Design review of the part built by this model. Coordinates are the model's own, in mm. A direction names the side the tool comes from. Give positions to 0.01 mm unless a question says otherwise; leave off trailing zeros. Loops run counter-clockwise (first coordinate to the right, second up) from the corner with the lowest first, then second, coordinate; pieces in that order, holes last. Notation, with made-up numbers: M -4.75,-22.75 L 8.25,-22.75 A21 ccw 8.25,3.25 Z; hole C 52,0.25 d5. An arc over 180 degrees is marked long. Use a Markdown table: item, result. Add a question column.
(1) Insertion check: pin 1 Ø3 at (x, y) = (-1, 56) entering from -Z; pin 2 Ø8 at (y, z) = (14.5, -5.5) entering from -X. Each pin has a flat end and moves straight along its axis. Give the tip position at first contact, or say it passes through.
(2) Add section B-B, the plane y = 42. Give the boundary of the cut face in (x, z).
(3) For faces 1 (the face through (-0.867, 31.798, 3.905)), 2 (the face through (-2.5, 67, 6)), list the 3-axis set-ups (+Z, -Z, +X, -X, +Y, -Y) from which the entire face can be reached by the end or side of a thin tool; tool diameter is ignored.
(4) Add section A-A, the plane z = -2.5. Give the boundary of the cut face in (x, y), then the cut area to 3 significant figures.
(5) Add section C-C, the plane z = 5.75. Give the boundary of the cut face in (x, y).
(6) For probe 1 along Z at (x, y) = (0.25, 23); probe 2 along Y at (x, z) = (-4.25, 2.75); probe 3 along X at (y, z) = (14, -0.5), list the stretches that pass through material, from the lowest coordinate up.
```python
from build123d import *

# Parameters (mm, degrees)
SKETCH1_R           = 4
BOSS_EXTRUDE1_DEPTH = 64.5
BOSS_EXTRUDE2_DEPTH = 5
CHAMFER1_SIZE       = 0.65


with BuildPart() as part:
    # Sketch1 → Boss-Extrude1 (new body)
    with BuildSketch(Plane(origin=(0, 0, 0), x_dir=(1, 0, 0), z_dir=(0, 1, 0))):
        Circle(SKETCH1_R)
    extrude(amount=BOSS_EXTRUDE1_DEPTH)

    # Sketch2 → Boss-Extrude2 (add)
    with BuildSketch(Plane(origin=(0, 64.5, 0), x_dir=(1, 0, 0), z_dir=(0, 1, 0))):
        Polygon((7.035549302, 0), (4.974884621, 4.974884621), (0, 7.035549302), (-4.974884621, 4.974884621), (-7.035549302, 0), (-4.974884621, -4.974884621), (0, -7.035549302), (4.974884621, -4.974884621), align=None)
    extrude(amount=BOSS_EXTRUDE2_DEPTH)

    # Chamfer1
    chamfer1_edges = [part.edges().sort_by_distance(p)[0] for p in [
        (-6.005216961, 69.5, 2.48744231),
        (-2.48744231, 69.5, 6.005216961),
        (2.48744231, 69.5, 6.005216961),
        (6.005216961, 64.5, 2.48744231),
        (6.005216961, 64.5, -2.48744231),
        (2.48744231, 64.5, -6.005216961),
        (-2.48744231, 64.5, -6.005216961),
        (-6.005216961, 64.5, -2.48744231),
        (-6.005216961, 64.5, 2.48744231),
        (-2.48744231, 64.5, 6.005216961),
        (2.48744231, 64.5, 6.005216961),
        (6.005216961, 69.5, 2.48744231),
        (6.005216961, 69.5, -2.48744231),
        (2.48744231, 69.5, -6.005216961),
        (-2.48744231, 69.5, -6.005216961),
        (-6.005216961, 69.5, -2.48744231),
    ]]
    chamfer(chamfer1_edges, length=CHAMFER1_SIZE)


solid = part.part
```
Established:
| question | item | result |
|---|---|---|
| 1 | pin 1 | z = -4 |
| 1 | pin 2 | x = -3.71 |
| 2 | outline | C 0,0 d8 |
| 3 | face 1 | -Y |
| 3 | face 2 | +Z, -X, +Y, -Y |
| 4 | outline | M -6,65.15 L -5.3,64.5 L -3.12,64.5 L -3.12,0 L 3.12,0 L 3.12,64.5 L 5.3,64.5 L 6,65.15 L 6,68.85 L 5.3,69.5 L -5.3,69.5 L -6,68.85 Z |
| 4 | area | 462 mm^2 |
| 5 | outline | M -3.1,65.15 L -1.41,64.5 L 1.41,64.5 L 3.1,65.15 L 3.1,68.85 L 1.41,69.5 L -1.41,69.5 L -3.1,68.85 Z |
| 6 | probe 1 | -3.99 to 3.99 |
| 6 | probe 2 | 64.5 to 69.5 |
| 6 | probe 3 | -3.97 to 3.97 |
